from build123d import *

# Parameters (mm, degrees)
BOX038_W                 = 6
BOX038_H                 = 42.4
BOX038_DEPTH             = 10.2
CYLINDER053_R            = 2
CYLINDER053_DEPTH        = 42
CYLINDER053_ROLL_ANGLE   = 90
PAD007_DEPTH             = 37
BODY008_PITCH_ANGLE      = -45
CYLINDER051_R            = 4
CYLINDER051_DEPTH        = 44
CYLINDER052_R            = 24
CYLINDER052_DEPTH        = 44
PAD006_DEPTH             = 5.62
PRISM012_DEPTH           = 20
PRISM012_PLACEMENT_ANGLE = 30
CHAMFER008_SIZE          = 10
THICKNESS001_T           = 3
CYLINDER055_R            = 1.5
CYLINDER055_DEPTH        = 15
BOX040_W                 = 4
BOX040_H                 = 7
BOX040_DEPTH             = 22
CHAMFER009_SIZE2         = 4
CHAMFER009_SIZE          = 15
BOX039_W                 = 12
BOX039_H                 = 10
BOX039_DEPTH             = 14
BOX039_ROLL_ANGLE        = -45
CYLINDER054_R            = 4
CYLINDER054_DEPTH        = 21
BOX041_W                 = 4
BOX041_H                 = 7
BOX041_DEPTH             = 10
CHAMFER010_SIZE          = 5
ARRAY003_COUNT           = 6


with BuildPart() as esfera:
    # Sphere → Sphere (revolve)
    with BuildSketch(Plane(origin=(-49, 0, 20), x_dir=(1, 0, 0), z_dir=(0, -1, 0))):
        with BuildLine():
            ThreePointArc((0, -7.5), (7.5, 0), (0, 7.5))
            Line((0, 7.5), (0, -7.5))
        make_face()
    revolve(axis=Axis((-49, 0, 20), (0, 0, 1)))


with BuildPart() as cubo034:
    # Box038 → Box038 (new body)
    with BuildSketch(Plane(origin=(44.7, -21.2, 0), x_dir=(1, 0, 0), z_dir=(0, 0, 1))):
        with Locations((3, 21.2)):
            Rectangle(BOX038_W, BOX038_H)
    extrude(amount=BOX038_DEPTH)


with BuildPart() as cylinder053:
    # Cylinder053 → Cylinder053 (new body)
    with BuildSketch(Plane.XY):
        Circle(CYLINDER053_R)
    extrude(amount=CYLINDER053_DEPTH)


with BuildPart() as cylinder053_1:
    # Cylinder053 roll: moved
    add(cylinder053.part.rotate(Axis((0, 0, 0), (1, 0, 0)), CYLINDER053_ROLL_ANGLE))


with BuildPart() as cylinder053_2:
    # Cylinder053 placement: moved
    add(cylinder053_1.part.moved(Location((-39, 21, 33))))


with BuildPart() as body008:
    # Sketch008 → Pad007 (new body)
    with BuildSketch(Plane.XY):
        Polygon((-40.876069, 10), (-49.536323, 5), (-49.536323, -5), (-40.876069, -10), (-32.215815, -5), (-32.215815, 5), align=None)
    extrude(amount=PAD007_DEPTH)


with BuildPart() as body008_1:
    # Body008 pitch: moved
    add(body008.part.rotate(Axis((0, 0, 0), (0, 1, 0)), BODY008_PITCH_ANGLE))


with BuildPart() as body008_2:
    # Body008 placement: moved
    add(body008_1.part.moved(Location((0, 0, 103))))


with BuildPart() as obj1:
    # Cylinder051 → Cylinder051 (new body)
    with BuildSketch(Plane(origin=(19, 7, 0), x_dir=(1, 0, 0), z_dir=(0, 0, 1))):
        Circle(CYLINDER051_R)
    extrude(amount=CYLINDER051_DEPTH)


with BuildPart() as fusion019:
    # Cylinder052 → Cylinder052 (new body)
    with BuildSketch(Plane.XY):
        Circle(CYLINDER052_R)
    extrude(amount=CYLINDER052_DEPTH)

    # Fusion019: union obj1
    add(obj1.part)


with BuildPart() as obj2:
    # Sketch007 → Pad006 (new body)
    with BuildSketch(Plane.YZ):
        Polygon((-3, 0.536587), (3, 0.536587), (4.5, -3.263413), (-4.5, -3.263413), align=None)
    extrude(amount=PAD006_DEPTH)


with BuildPart() as obj2_1:
    # Body007 placement: moved
    add(obj2.part.moved(Location((45.85, 0, 5))))


with BuildPart() as superior001:
    # Prism012 → Prism012 (new body)
    with BuildSketch(Plane.XY):
        Polygon((55, 0), (27.5, 47.631397), (-27.5, 47.631397), (-55, 0), (-27.5, -47.631397), (27.5, -47.631397), align=None)
    extrude(amount=PRISM012_DEPTH)


with BuildPart() as superior001_1:
    # Prism012 placement: moved
    add(superior001.part.rotate(Axis((0, 0, 0), (0, 0, 1)), PRISM012_PLACEMENT_ANGLE))

    # Chamfer008
    chamfer008_edges = [superior001_1.edges().sort_by_distance(p)[0] for p in [
        (23.815699, 41.25, 20),
        (-23.815699, 41.25, 20),
        (-47.631397, 0, 20),
        (-23.815699, -41.25, 20),
        (23.815699, -41.25, 20),
        (47.631397, 0, 20),
    ]]
    chamfer(chamfer008_edges, length=CHAMFER008_SIZE)

    # Thickness001
    thickness001_openings = [superior001_1.faces().sort_by_distance(p)[0] for p in [
        (0, 0, 0),
    ]]
    offset(amount=THICKNESS001_T, openings=thickness001_openings, kind=Kind.INTERSECTION)

    # Cut022: cut obj2
    add(obj2_1.part, mode=Mode.SUBTRACT)

    # Cut023: cut Fusion019
    add(fusion019.part, mode=Mode.SUBTRACT)

    # Cut024: cut Body008
    add(body008_2.part, mode=Mode.SUBTRACT)

    # Cut025: cut Cylinder053
    add(cylinder053_2.part, mode=Mode.SUBTRACT)

    # Cut026: cut Cubo034
    add(cubo034.part, mode=Mode.SUBTRACT)


with BuildPart() as cilindro028:
    # Cylinder055 → Cylinder055 (new body)
    with BuildSketch(Plane(origin=(0, -46, 0), x_dir=(1, 0, 0), z_dir=(0, 0, 1))):
        Circle(CYLINDER055_R)
    extrude(amount=CYLINDER055_DEPTH)


with BuildPart() as chamfer009:
    # Box040 → Box040 (new body)
    with BuildSketch(Plane(origin=(-2, -43, 0), x_dir=(1, 0, 0), z_dir=(0, 0, 1))):
        with Locations((2, 3.5)):
            Rectangle(BOX040_W, BOX040_H)
    extrude(amount=BOX040_DEPTH)

    # Chamfer009
    chamfer009_edges = [chamfer009.edges().sort_by_distance(p)[0] for p in [
        (0, -36, 0),
    ]]
    chamfer009_side = chamfer009.faces().sort_by_distance((0, -36, 11))[0]
    chamfer(chamfer009_edges, length=CHAMFER009_SIZE, length2=CHAMFER009_SIZE2, reference=chamfer009_side)


with BuildPart() as cubo035:
    # Box039 → Box039 (new body)
    with BuildSketch(Plane.XY):
        with Locations((6, 5)):
            Rectangle(BOX039_W, BOX039_H)
    extrude(amount=BOX039_DEPTH)


with BuildPart() as cubo035_1:
    # Box039 roll: moved
    add(cubo035.part.rotate(Axis((0, 0, 0), (1, 0, 0)), BOX039_ROLL_ANGLE))


with BuildPart() as cubo035_2:
    # Box039 placement: moved
    add(cubo035_1.part.moved(Location((-7, -59, 20))))


with BuildPart() as cut027:
    # Cylinder054 → Cylinder054 (new body)
    with BuildSketch(Plane(origin=(0, -46, 0), x_dir=(1, 0, 0), z_dir=(0, 0, 1))):
        Circle(CYLINDER054_R)
    extrude(amount=CYLINDER054_DEPTH)

    # Cut027: cut Cubo035
    add(cubo035_2.part, mode=Mode.SUBTRACT)


with BuildPart() as superior_final:
    # Box041 → Box041 (new body)
    with BuildSketch(Plane(origin=(-2, -56, 6), x_dir=(1, 0, 0), z_dir=(0, 0, 1))):
        with Locations((2, 3.5)):
            Rectangle(BOX041_W, BOX041_H)
    extrude(amount=BOX041_DEPTH)

    # Chamfer010
    chamfer010_edges = [superior_final.edges().sort_by_distance(p)[0] for p in [
        (0, -56, 16),
    ]]
    chamfer(chamfer010_edges, length=CHAMFER010_SIZE)

    # Fusion020: union Chamfer009, Cut027
    add(chamfer009.part)
    add(cut027.part)

    # Cut028: cut Cilindro028
    add(cilindro028.part, mode=Mode.SUBTRACT)

    # Array003: superior final ×6 about axis
    array003_axis = Axis((0, 0, 0), (0, 0, 1))


with BuildPart() as superior_final_1:
    add(superior_final.part)
    for i in range(1, ARRAY003_COUNT):
        add(superior_final.part.rotate(array003_axis, i * 360 / ARRAY003_COUNT))

    # Fusion021: union superior001
    add(superior001_1.part)

    # Cut029: cut Esfera
    add(esfera.part, mode=Mode.SUBTRACT)


solid = superior_final_1.part
Here's how the part is built. I have some questions about the finished solid (model axes, mm). A direction names the side the tool comes from. Round coordinates to 2 decimals unless told otherwise and drop trailing zeros. Order: outer loops, then holes, each group sorted by start corner. A loop starts at its lowest first (then second) coordinate and runs counter-clockwise, first axis right, second up. Notation, with made-up numbers: (27.25, 62.5) -> (70.25, 62.5) arc R16 ccw to (70.25, 70.5) -> close; hole circle Ø11 at (-32, 21). An arc over 180 degrees is marked (long way). Use CSV: the item, a comma, the result in double quotes.
1. I need wall thicknesses on line 1 along Y through (x, z) = (35.5, 8.75); line 2 along Y through (x, z) = (-33.5, 19.5); line 3 along Z through (x, y) = (19, 17.5). Which ranges of each line are inside material? Lowest first, please.
Recorded:
line 1,"y = -37.97 to -34.5, -22.81 to -18.19, 18.19 to 22.81, 34.5 to 37.97"
line 2,"y = -29.59 to -24.69, -21.65 to -17.03, 17.03 to 21.65, 24.69 to 29.59"
line 3,"z = 20 to 23"
2. I want a section at D-D on y = -33. List the corners of the cut face in (x, z) for me.
Recorded:
outline,"(-44.11, 0) -> (-38.11, 0) -> (-38.11, 10) -> (-18.11, 20) -> (18.11, 20) -> (38.11, 10) -> (38.11, 0) -> (44.11, 0) -> (44.11, 11.24) -> (20.59, 23) -> (-20.59, 23) -> (-44.11, 11.24) -> close"
3. Thinking about a two-plate mould opening in X: for faces 1 (the face through (0, -44, 0)), 2 (the face through (-35.7, 18.3, 12.1)), 3 (the face through (-25.67, -43.643, 5.543)), which applies, pulls with the +X half, pulls with the -X half, needs draft (parallel to the pull), parting line crosses it, or undercut?
Recorded:
face 1,"needs draft"
face 2,"undercut"
face 3,"pulls with the -X half"
4. I want a section at C-C on z = 4.5. Give the number of separate pieces and of enclosed holes in the cut face, and give its area (3 significant figures).
Recorded:
separate pieces,"7"
enclosed holes,"6"
area,"1,230 mm2"
5. I want a section at A-A on x = 9. List the corners of the cut face in (y, z) for me.
Recorded:
outline,"(-53.27, 0) -> (-49.8, 0) -> (-49.8, 10) -> (-38.26, 20) -> (-22.25, 20) -> (-22.25, 23) -> (-39.69, 23) -> (-53.27, 11.24) -> close; (22.25, 20) -> (38.26, 20) -> (49.8, 10) -> (49.8, 0) -> (53.27, 0) -> (53.27, 11.24) -> (39.69, 23) -> (22.25, 23) -> close"
6. I'm going to push flat-ended pins straight in: P1, Ø1.2, axis at x = 1, y = -51.5, coming from the -Z side; P2, Ø1.5, axis at x = -0.5, y = -45.5, coming from the -Z side; P3, Ø11, axis at y = -3, z = 4, coming from the +X side. Where does each tip first touch, or does it pass through?
Recorded:
P1,"stops at z = 6"
P2,"stops at z = 15"
P3,"stops at x = -47.63"
7. Which directions (+Z, -Z, +X, -X, +Y, -Y) give clear straight access to the entire face, cutting with the end or side of a thin tool? Please do faces 4 (the face through (33.676, 21.752, 12.082)), 5 (the face through (-22.69, -38.481, 17.204)).
Recorded:
face 4,"-Z"
face 5,"+Z, -X, -Y"
8. I want a section at B-B on y = -11.5. List the corners of the cut face in (x, z) for me.
Recorded:
outline,"(-50.63, 0) -> (-47.63, 0) -> (-47.63, 10) -> (-37.63, 20) -> (-21.07, 20) -> (-21.07, 23) -> (-38.87, 23) -> (-50.63, 11.24) -> close; (21.07, 20) -> (37.63, 20) -> (47.43, 10.2) -> (50.63, 10.2) -> (50.63, 11.24) -> (38.87, 23) -> (21.07, 23) -> close"
